```python
from build123d import *

# Parameters (mm, degrees)
SALIENTE_EXTRUIR2_DEPTH = 100
CROQUIS2_W              = 110
CROQUIS2_H              = 110
SALIENTE_EXTRUIR3_DEPTH = 5
CROQUIS3_W              = 110
CROQUIS3_H              = 110
SALIENTE_EXTRUIR4_DEPTH = 5
CROQUIS4_W              = 90
CROQUIS4_H              = 90
SALIENTE_EXTRUIR5_DEPTH = 5
CROQUIS5_W              = 50
CROQUIS5_H              = 50
SALIENTE_EXTRUIR6_DEPTH = 5
CROQUIS6_W              = 10
CROQUIS6_H              = 10
SALIENTE_EXTRUIR7_DEPTH = 25
CROQUIS7_W              = 30
CROQUIS7_H              = 10
SALIENTE_EXTRUIR8_DEPTH = 5


with BuildPart() as part:
    # Croquis1 → Saliente-Extruir2 (new body)
    with BuildSketch(Plane.XY):
        Polygon((-45, 50), (45, 50), (45, 55), (55, 55), (55, 45), (50, 45), (50, -45), (55, -45), (55, -55), (45, -55), (45, -50), (-45, -50), (-45, -55), (-55, -55), (-55, -45), (-50, -45), (-50, 45), (-55, 45), (-55, 55), (-45, 55), align=None)
    extrude(amount=SALIENTE_EXTRUIR2_DEPTH)

    # Croquis2 → Saliente-Extruir3 (add)
    with BuildSketch(Plane.XY.offset(100)):
        Rectangle(CROQUIS2_W, CROQUIS2_H)
    extrude(amount=SALIENTE_EXTRUIR3_DEPTH)

    # Croquis3 → Saliente-Extruir4 (add)
    with BuildSketch(Plane(origin=(0, 0, 0), x_dir=(-1, 0, 0), z_dir=(0, 0, -1))):
        Rectangle(CROQUIS3_W, CROQUIS3_H)
    extrude(amount=SALIENTE_EXTRUIR4_DEPTH)

    # Croquis4 → Saliente-Extruir5 (add)
    with BuildSketch(Plane.XY.offset(105)):
        Rectangle(CROQUIS4_W, CROQUIS4_H)
    extrude(amount=SALIENTE_EXTRUIR5_DEPTH)

    # Croquis5 → Saliente-Extruir6 (add)
    with BuildSketch(Plane.XY.offset(110)):
        Rectangle(CROQUIS5_W, CROQUIS5_H)
    extrude(amount=SALIENTE_EXTRUIR6_DEPTH)

    # Croquis6 → Saliente-Extruir7 (add)
    with BuildSketch(Plane.XY.offset(115)):
        with Locations((-10, -0.15538451)):
            Rectangle(CROQUIS6_W, CROQUIS6_H)
        with Locations((10, -0.15538451)):
            Rectangle(CROQUIS6_W, CROQUIS6_H)
    extrude(amount=SALIENTE_EXTRUIR7_DEPTH)

    # Croquis7 → Saliente-Extruir8 (add)
    with BuildSketch(Plane.XY.offset(140)):
        with Locations((0, -0.15538451)):
            Rectangle(CROQUIS7_W, CROQUIS7_H)
    extrude(amount=SALIENTE_EXTRUIR8_DEPTH)


solid = part.part
```
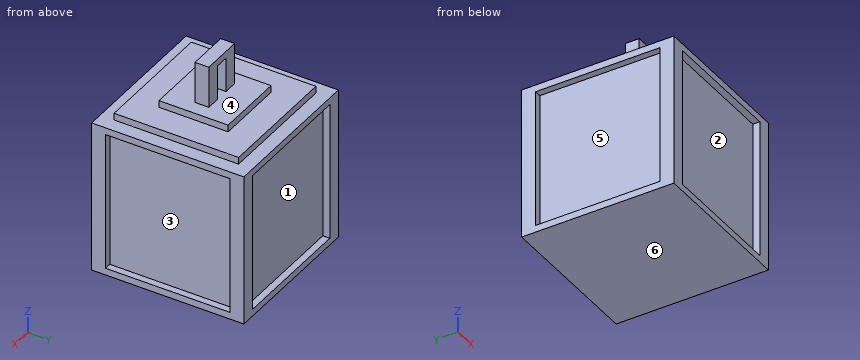
Can you work these out from the model? Positions are in its coordinate system, mm. Face numbers are marked on the shaded views. A direction names the side the tool comes from. Round coordinates to 2 decimals unless told otherwise and drop trailing zeros. Order: outer loops, then holes, each group sorted by start corner. A loop starts at its lowest first (then second) coordinate and runs counter-clockwise, first axis right, second up. Notation, with made-up numbers: (66.25, 73) -> (74.25, 73) arc R20 cw to (74.25, 110) -> close; hole circle Ø8 at (73, 45.5). An arc over 180 degrees is marked (long way). Return JSON: item names as keys, results as strings. Group by question number.
1. If we section it at A-A, the plane z = 127: Write out the boundary of the cut face in (x, y), then the cut area to 3 significant figures.
2. We'd pull the mould along Y, two halves only. Please class the marked faces 1, 2, 3 and 4: released by +Y, released by -Y, zero draft, split by the parting line, or undercut.
3. Will these pins go through, and if not, where does the flat tip stop? pin 1 (4 mm diameter, centred on y = -24, z = 46.5, fed in from +X); pin 2 (4 mm diameter, centred on x = -8, y = -53, fed in from +Z); pin 3 (2 mm diameter, centred on y = 7.5, z = 68.5, fed in from -X).
4. If we section it at D-D, the plane z = 57: Write out the boundary of the cut face in (x, y), then the cut area to 3 significant figures.
5. Which directions (+Z, -Z, +X, -X, +Y, -Y) give clear straight access to the entire face, cutting with the end or side of a thin tool? Please do the marked faces 5 and 6.
6. I need wall thicknesses on line 1 (Z direction, x = 51.5, y = -23); line 2 (Z direction, x = 38, y = -38); line 3 (Y direction, x = -39.5, z = 19). Which ranges of each line are inside material? Lowest first, please. Write a range as [from, to].
7. If we section it at C-C, the plane y = 27: Write out the boundary of the cut face in (x, z).
8. If we section it at B-B, the plane x = 1: Write out the boundary of the cut face in (y, z), then the cut area to 4 significant figures.
Output values:
{
 "1": {"outline": "(-15, -5.16) -> (-5, -5.16) -> (-5, 4.84) -> (-15, 4.84) -> close; (5, -5.16) -> (15, -5.16) -> (15, 4.84) -> (5, 4.84) -> close", "area": "200 mm²"},
 "2": {"face 1": "released by +Y", "face 2": "released by -Y", "face 3": "undercut", "face 4": "zero draft"},
 "3": {"pin 1": "x = 50", "pin 2": "z = 105", "pin 3": "x = -50"},
 "4": {"outline": "(-55, -55) -> (-45, -55) -> (-45, -50) -> (45, -50) -> (45, -55) -> (55, -55) -> (55, -45) -> (50, -45) -> (50, 45) -> (55, 45) -> (55, 55) -> (45, 55) -> (45, 50) -> (-45, 50) -> (-45, 55) -> (-55, 55) -> (-55, 45) -> (-50, 45) -> (-50, -45) -> (-55, -45) -> close", "area": "10,300 mm²"},
 "5": {"face 5": "-X", "face 6": "-Z, +X, -X, +Y, -Y"},
 "6": {"line 1": "[-5, 0], [100, 105]", "line 2": "[-5, 110]", "line 3": "[-50, 50]"},
 "7": {"outline": "(-55, -5) -> (55, -5) -> (55, 0) -> (50, 0) -> (50, 100) -> (55, 100) -> (55, 105) -> (45, 105) -> (45, 110) -> (-45, 110) -> (-45, 105) -> (-55, 105) -> (-55, 100) -> (-50, 100) -> (-50, 0) -> (-55, 0) -> close"},
 "8": {"outline": "(-55, -5) -> (55, -5) -> (55, 0) -> (50, 0) -> (50, 100) -> (55, 100) -> (55, 105) -> (45, 105) -> (45, 110) -> (25, 110) -> (25, 115) -> (-25, 115) -> (-25, 110) -> (-45, 110) -> (-45, 105) -> (-55, 105) -> (-55, 100) -> (-50, 100) -> (-50, 0) -> (-55, 0) -> close; (-5.16, 140) -> (4.84, 140) -> (4.84, 145) -> (-5.16, 145) -> close", "area": "11,850 mm²"}
}
